The listing builds one solid part. Answer for the finished solid, in the listing's coordinates (mm). A direction names the side the tool comes from. Give positions to 0.01 mm unless a question says otherwise; leave off trailing zeros. Order: outer loops, then holes, each group sorted by start corner. A loop starts at its lowest first (then second) coordinate and runs counter-clockwise, first axis right, second up. Notation, with made-up numbers: (6, -22) - (25, -22) arc R17 ccw to (25, -2) - close; hole circle Ø4 at (-20, -27). An arc over 180 degrees is marked (long way). Use CSV: the item, a comma, the result in double quotes.
```python
from build123d import *

# Parameters (mm, degrees)
SKETCH1_W            = 20
SKETCH1_H            = 50
BOSS_EXTRUDE1_DEPTH  = 10
SKETCH5_W            = 19.05
SKETCH5_H            = 19.05
CUT_EXTRUDE1_DEPTH   = 6.35
SKETCH7_W            = 20
SKETCH7_H            = 50
BOSS_EXTRUDE2_DEPTH  = 35
M4_CLEARANCE_HOLE1_D = 4.3


with BuildPart() as part:
    # Sketch1 → Boss-Extrude1 (new body)
    with BuildSketch(Plane(origin=(0, 0, 0), x_dir=(0, 0, -1), z_dir=(1, 0, 0))):
        with Locations((-10, 0)):
            Rectangle(SKETCH1_W, SKETCH1_H)
        with BuildLine():
            ThreePointArc((25.466783574, 8.373426859), (30, 0), (25.466783574, -8.373426859))
            Line((25.466783574, -8.373426859), (0, -25))
            Line((0, -25), (0, 25))
            Line((0, 25), (25.466783574, 8.373426859))
        make_face()
    extrude(amount=BOSS_EXTRUDE1_DEPTH)

    # Sketch5 → Cut-Extrude1 (cut)
    with BuildSketch(Plane(origin=(10, 0, 0), x_dir=(0, 0, -1), z_dir=(1, 0, 0))):
        with Locations((-4.915565879, 0)):
            Rectangle(SKETCH5_W, SKETCH5_H)
    extrude(amount=-CUT_EXTRUDE1_DEPTH, mode=Mode.SUBTRACT)

    # Sketch7 → Boss-Extrude2 (add)
    with BuildSketch(Plane.ZY):
        with Locations((10, 0)):
            Rectangle(SKETCH7_W, SKETCH7_H)
    extrude(amount=BOSS_EXTRUDE2_DEPTH)

    # M4 Clearance Hole1 (through all)
    with Locations(Plane.XY.offset(20)):
        with Locations((-25, 20), (-25, -10), (-5, 5)):
            Hole(M4_CLEARANCE_HOLE1_D / 2)


solid = part.part
```
Item 1: Find the intervals of material crossed by line 1 along Y through (x, z) = (-25, 5); line 2 along Y through (x, z) = (-5, 4); line 3 along Z through (x, y) = (-32.5, -15.5), in increasing order.
Taken from the geometry:
line 1,"-25 to -12.15, -7.85 to 17.85, 22.15 to 25"
line 2,"-25 to 2.85, 7.15 to 25"
line 3,"0 to 20"
Item 2: The part is cut by section C-C (y = 5). Give the vertices of the cut face in (x, z).
Taken from the geometry:
outline,"(-35, 0) - (-7.15, 0) - (-7.15, 20) - (-35, 20) - close; (-2.85, 0) - (0, 0) - (0, -28.66) - (10, -28.66) - (10, -4.61) - (3.65, -4.61) - (3.65, 14.44) - (10, 14.44) - (10, 20) - (-2.85, 20) - close"
Item 3: The mould has two halves that part along Y. Classify faces 4 (the face through (4.93, -16.57, -12.91)), 5 (the face through (10, 0, -5)), 6 (the face through (7, 9.525, 5)): +Y half, -Y half, draft (parallel to the pull), parting line (faces both ways), or undercut.
Taken from the geometry:
face 4,"-Y half"
face 5,"draft"
face 6,"undercut"
Item 4: Which of the six approach directions +Z, -Z, +X, -X, +Y, -Y give full straight-line access (tool end or side, diameter ignored) to faces 1 (the face through (0, 0, -11)), 2 (the face through (-35, 0, 10)), 3 (the face through (7, -9.525, 5))?
Taken from the geometry:
face 1,"-Z, -X, +Y, -Y"
face 2,"+Z, -Z, -X, +Y, -Y"
face 3,"+X"
Item 5: The part is cut by section B-B (z = 16). Give the vertices of the cut face in (x, y).
Taken from the geometry:
outline,"(-35, -25) - (10, -25) - (10, 25) - (-35, 25) - close; hole circle Ø4.3 at (-25, -10); hole circle Ø4.3 at (-25, 20); hole circle Ø4.3 at (-5, 5)"
Item 6: The part is cut by section A-A (x = -25). Give the vertices of the cut face in (y, z).
Taken from the geometry:
outline,"(-25, 0) - (-12.15, 0) - (-12.15, 20) - (-25, 20) - close; (-7.85, 0) - (17.85, 0) - (17.85, 20) - (-7.85, 20) - close; (22.15, 0) - (25, 0) - (25, 20) - (22.15, 20) - close"
Item 7: The part is cut by section D-D (x = -5). Give the vertices of the cut face in (y, z), and give its area (3 significant figures).
Taken from the geometry:
outline,"(-25, 0) - (2.85, 0) - (2.85, 20) - (-25, 20) - close; (7.15, 0) - (25, 0) - (25, 20) - (7.15, 20) - close"
area,"914 mm^2"
Item 8: Each of these flat-tipped pins is pushed along its axis until it touches: pin 1 (9 mm diameter, centred on y = -11.5, z = -21, fed in from -X); pin 2 (7 mm diameter, centred on x = -25, y = -10, fed in from -Z). Where does it stop, or does it pass through?
Taken from the geometry:
pin 1,"x = 0"
pin 2,"z = 0"
